```python
from build123d import *

# Parameters (mm, degrees)
SKETCH1_W                                      = 144
SKETCH1_H                                      = 20
BOSS_EXTRUDE1_DEPTH                            = 6
CSK_FOR_M5_FLAT_HEAD_MACHINE_SCREW1_AT_2_COUNT = 2
CSK_FOR_M5_FLAT_HEAD_MACHINE_SCREW1_AT_2_PITCH = 70


with BuildPart() as part:
    # Sketch1 → Boss-Extrude1 (new body)
    with BuildSketch(Plane(origin=(0, 0, 0), x_dir=(1, 0, 0), z_dir=(0, 1, 0))):
        with Locations((72, 10)):
            Rectangle(SKETCH1_W, SKETCH1_H)
    extrude(amount=BOSS_EXTRUDE1_DEPTH)

    # Sketch2 → CSK for M5 Flat Head Machine Screw1 (revolve, cut)
    with BuildSketch(Plane(origin=(38, 6, -10), x_dir=(0, 0, 1), z_dir=(1, 0, 0))):
        Polygon((0, 0), (0, 6), (3.5, 6), (3.5, 3.575260778), (6.5, 0), align=None)
    csk_for_m5_flat_head_machine_screw1 = revolve(axis=Axis((38, 12.35, -10), (0, -1, 0)), mode=Mode.SUBTRACT)

    # CSK for M5 Flat Head Machine Screw1 at 2: CSK for M5 Flat Head Machine Screw1 ×2
    with Locations(*[(i * CSK_FOR_M5_FLAT_HEAD_MACHINE_SCREW1_AT_2_PITCH, 0, 0) for i in range(1, CSK_FOR_M5_FLAT_HEAD_MACHINE_SCREW1_AT_2_COUNT)]):
        add(csk_for_m5_flat_head_machine_screw1, mode=Mode.SUBTRACT)


solid = part.part
```
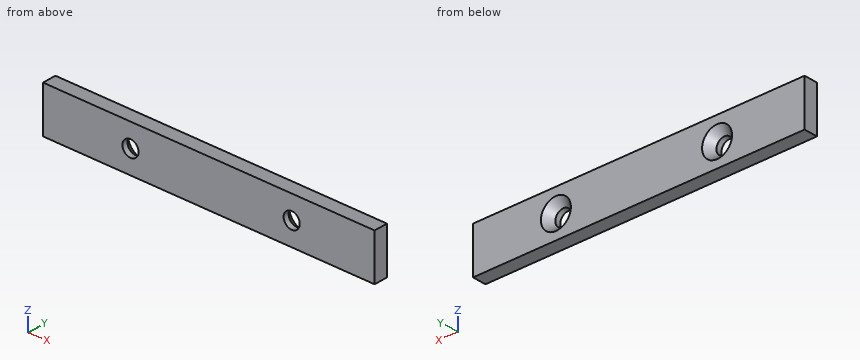
Geometry check sheet. Reference: the model listing, model coordinates, mm. Round coordinates to 2 decimals unless told otherwise and drop trailing zeros. Loops run counter-clockwise (first coordinate to the right, second up) from the corner with the lowest first, then second, coordinate; pieces in that order, holes last. Notation, with made-up numbers: (82.25, -32.75) -> (140.25, -32.75) arc R12 ccw to (140.25, -23.75) -> close; hole circle Ø11 at (50, 33). An arc over 180 degrees is marked (long way). Use a Markdown table: item, result.
(1) Sectioned sample at C-C (y = 4.95). Enter the section's corners in (x, z), then the cut area to 3 significant figures.
Calculated:
| item | result |
|---|---|
| outline | (0, -20) -> (144, -20) -> (144, 0) -> (0, 0) -> close; hole circle Ø11.24 at (38, -10); hole circle Ø11.24 at (108, -10) |
| area | 2,680 mm² |
(2) Sectioned sample at B-B (x = 108). Enter the section's corners in (y, z), then the cut area to 3 significant figures.
Calculated:
| item | result |
|---|---|
| outline | (0, -20) -> (6, -20) -> (6, -16.5) -> (2.42, -13.5) -> (0, -13.5) -> close; (0, -6.5) -> (2.42, -6.5) -> (6, -3.5) -> (6, 0) -> (0, 0) -> close |
| area | 67.3 mm² |
(3) Go/stop test with flat-tipped pins: P1, Ø8, axis at x = 38, z = -10, coming from the +Y side; P2, Ø3, axis at x = 18, z = -14.5, coming from the -Y side. Record where each tip stops, or that it passes through.
Calculated:
| item | result |
|---|---|
| P1 | y = 3.02 |
| P2 | y = 0 |
(4) Sectioned sample at A-A (z = -10). Enter the section's corners in (x, y).
Calculated:
| item | result |
|---|---|
| outline | (0, 0) -> (34.5, 0) -> (34.5, 2.42) -> (31.5, 6) -> (0, 6) -> close; (41.5, 0) -> (104.5, 0) -> (104.5, 2.42) -> (101.5, 6) -> (44.5, 6) -> (41.5, 2.42) -> close; (111.5, 0) -> (144, 0) -> (144, 6) -> (114.5, 6) -> (111.5, 2.42) -> close |
(5) Scan lines: probe 1 along X at (y, z) = (1.6, -10); probe 2 along Z at (x, y) = (38, 0.5); probe 3 along X at (y, z) = (3.9, -8.5). Record each from-to range of solid material in increasing order.
Calculated:
| item | result |
|---|---|
| probe 1 | 0 to 34.5, 41.5 to 104.5, 111.5 to 144 |
| probe 2 | -20 to -13.5, -6.5 to 0 |
| probe 3 | 0 to 33.51, 42.49 to 103.51, 112.49 to 144 |
